Verification items for this drawing (mm, ordinates from the low corner). A direction names the side the tool comes from. Give positions to 0.01 mm unless a question says otherwise; leave off trailing zeros. Loops run counter-clockwise (first coordinate to the right, second up) from the corner with the lowest first, then second, coordinate; pieces in that order, holes last. Notation, with made-up numbers: M 47,28.5 L 89,28.5 A21 cw 89,37.5 Z; hole C 24,-36 d11. An arc over 180 degrees is marked long. Use a Markdown table: item, result.
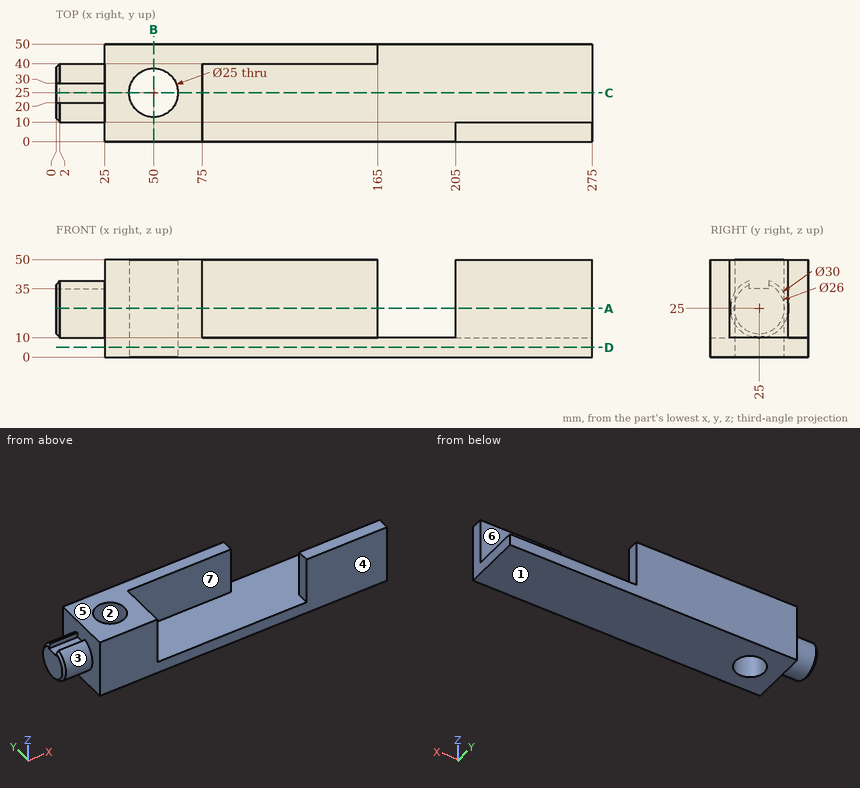
(1) Cross-section at A-A on z = 25. Record the cut outline in (x, y), then the cut area to 3 significant figures.
Results below:
| item | result |
|---|---|
| outline | M 0,12 L 2,10 L 25,10 L 25,0 L 75,0 L 75,40 L 165,40 L 165,50 L 25,50 L 25,40 L 2,40 L 0,38 Z; M 205,0 L 275,0 L 275,10 L 205,10 Z; hole C 50,25 d25 |
| area | 4,360 mm^2 |
(2) Gauge pin test, flat ends, axial feed: P1, Ø2, axis at x = 154.5, y = 13.5, coming from the -Z side; P2, Ø4, axis at y = 6.5, z = 27, coming from the -X side; P3, Ø5, axis at x = 10, y = 25.5, coming from the +Z side; P4, Ø3.5, axis at x = 15.5, z = 36, coming from the -Y side. Record the tip position at first contact, or that the pin passes through.
Results below:
| item | result |
|---|---|
| P1 | z = 0 |
| P2 | x = 25 |
| P3 | z = 35 |
| P4 | y = 13.19 |
(3) Cross-section at D-D on z = 5. Record the cut outline in (x, y).
Results below:
| item | result |
|---|---|
| outline | M 25,0 L 275,0 L 275,50 L 25,50 Z; hole C 50,25 d25 |
(4) Draft check along Y on the marked faces 1, 2, 3 and 4. Enter one of: +Y half, -Y half, draft (parallel to the pull), parting line (faces both ways), or undercut.
Results below:
| item | result |
|---|---|
| face 1 | draft |
| face 2 | undercut |
| face 3 | parting line |
| face 4 | -Y half |
(5) Cross-section at C-C on y = 25. Record the cut outline in (x, z), then the cut area to 3 significant figures.
Results below:
| item | result |
|---|---|
| outline | M 0,12 L 2,10 L 25,10 L 25,0 L 37.5,0 L 37.5,50 L 25,50 L 25,35 L 0,35 Z; M 62.5,0 L 275,0 L 275,10 L 75,10 L 75,50 L 62.5,50 Z |
| area | 3,870 mm^2 |
(6) Set-up check for the marked faces 5, 6 and 7: record each of +Z, -Z, +X, -X, +Y, -Y from which the full face is reachable in a straight line by a thin tool's end or side.
Results below:
| item | result |
|---|---|
| face 5 | +Z, +X, -X, +Y, -Y |
| face 6 | +Z, +X, +Y |
| face 7 | +Z, +X, -Y |
(7) Cross-section at B-B on x = 50. Record the cut outline in (y, z), then the cut area to 3 significant figures.
Results below:
| item | result |
|---|---|
| outline | M 0,0 L 12.5,0 L 12.5,50 L 0,50 Z; M 37.5,0 L 50,0 L 50,50 L 37.5,50 Z |
| area | 1,250 mm^2 |
(8) Material ranges on line 1 (Y direction, x = 50, z = 24.5); line 2 (X direction, y = 4.5, z = 29.5); line 3 (X direction, y = 12, z = 12.5), recorded low to high.
Results below:
| item | result |
|---|---|
| line 1 | 0 to 12.5, 37.5 to 50 |
| line 2 | 25 to 75, 205 to 275 |
| line 3 | 25 to 75 |
